```python
from build123d import *

# Parameters (mm, degrees)
F1_DEPTH = 7.5
F3_DEPTH = 5
F5_R     = 0.8
F6_DEPTH = 45


# Not quite as in the source:
# - ends of sketch curves that miss each other by under 0.0002 mm in the source are joined
# - a feature names something its author has since deleted; it is built from what else it names


with BuildPart() as f1:
    # F0 (on Right) → F1 (new body)
    with BuildSketch(Plane.YZ):
        with BuildLine():
            ThreePointArc((9.2226032736, 0.0929824566), (9.0820111575, -0.0673321366), (8.8773, -0.127))
            Line((8.8773, -0.127), (6.3627, -0.127))
            ThreePointArc((6.3627, -0.127), (6.1579888425, -0.0673321366), (6.0173967264, 0.0929824566))
            Line((6.0173967264, 0.0929824566), (5.6288146574, 0.9262855682))
            ThreePointArc((5.6288146574, 0.9262855682), (5.4882390894, 1.0842993961), (5.2850542, 1.143))
            Line((5.2850542, 1.143), (4.8749458, 1.143))
            ThreePointArc((4.8749458, 1.143), (4.668712979, 1.0823576494), (4.5281307776, 0.9197350317))
            Line((4.5281307776, 0.9197350317), (4.1426086033, 0.0929799713))
            ThreePointArc((4.1426086033, 0.0929799713), (4.0020111575, -0.0673321366), (3.7973, -0.127))
            Line((3.7973, -0.127), (1.2827, -0.127))
            ThreePointArc((1.2827, -0.127), (1.0779888425, -0.0673321366), (0.9373967264, 0.0929824566))
            Line((0.9373967264, 0.0929824566), (0.5488146574, 0.9262855682))
            ThreePointArc((0.5488146574, 0.9262855682), (0.4082390894, 1.0842993961), (0.2050542, 1.143))
            Line((0.2050542, 1.143), (-0.2050542, 1.143))
            ThreePointArc((-0.2050542, 1.143), (-0.411287021, 1.0823576494), (-0.5518692224, 0.9197350317))
            Line((-0.5518692224, 0.9197350317), (-0.9373913967, 0.0929799713))
            ThreePointArc((-0.9373913967, 0.0929799713), (-1.0779888425, -0.0673321366), (-1.2827, -0.127))
            Line((-1.2827, -0.127), (-3.7973, -0.127))
            ThreePointArc((-3.7973, -0.127), (-4.0020111575, -0.0673321366), (-4.1426032736, 0.0929824566))
            Line((-4.1426032736, 0.0929824566), (-4.5311853426, 0.9262855682))
            ThreePointArc((-4.5311853426, 0.9262855682), (-4.6717609106, 1.0842993961), (-4.8749458, 1.143))
            Line((-4.8749458, 1.143), (-5.2850542, 1.143))
            ThreePointArc((-5.2850542, 1.143), (-5.491287021, 1.0823576494), (-5.6318692224, 0.9197350317))
            Line((-5.6318692224, 0.9197350317), (-6.0173913967, 0.0929799713))
            ThreePointArc((-6.0173913967, 0.0929799713), (-6.1579888425, -0.0673321366), (-6.3627, -0.127))
            Line((-6.3627, -0.127), (-8.8773, -0.127))
            ThreePointArc((-8.8773, -0.127), (-9.0820111575, -0.0673321366), (-9.2226032736, 0.0929824566))
            Line((-9.2226032736, 0.0929824566), (-9.6111853426, 0.9262855682))
            ThreePointArc((-9.6111853426, 0.9262855682), (-9.7517609106, 1.0842993961), (-9.9549458, 1.143))
            Line((-9.9549458, 1.143), (-10.3650542, 1.143))
            ThreePointArc((-10.3650542, 1.143), (-10.571287021, 1.0823576494), (-10.7118692224, 0.9197350317))
            Line((-10.7118692224, 0.9197350317), (-11.0973913967, 0.0929799713))
            ThreePointArc((-11.0973913967, 0.0929799713), (-11.2379888425, -0.0673321366), (-11.4427, -0.127))
            Line((-11.4427, -0.127), (-12.7, -0.127))
            Line((-12.7, -0.127), (-12.7, -1.143))
            Line((-12.7, -1.143), (12.7, -1.143))
            Line((12.7, -1.143), (12.7, -0.127))
            Line((12.7, -0.127), (11.4427, -0.127))
            ThreePointArc((11.4427, -0.127), (11.2379888425, -0.0673321366), (11.0973967264, 0.0929824566))
            Line((11.0973967264, 0.0929824566), (10.7088146574, 0.9262855682))
            ThreePointArc((10.7088146574, 0.9262855682), (10.5682390894, 1.0842993961), (10.3650542, 1.143))
            Line((10.3650542, 1.143), (9.9549458, 1.143))
            ThreePointArc((9.9549458, 1.143), (9.748712979, 1.0823576494), (9.6081307776, 0.9197350317))
            Line((9.6081307776, 0.9197350317), (9.2226032736, 0.0929824566))
        make_face()
    extrude(amount=-F1_DEPTH)

    # F2 (on face) → F3 (join)
    with BuildSketch(Plane(origin=(-7.5, 0, 0), x_dir=(0, -1, 0), z_dir=(-1, 0, 0))):
        Polygon((-11.4427, -0.127), (-12.7, -0.127), (-12.7, -1.143), (12.7, -1.143), (12.7, -0.127), (11.4427, -0.127), (8.8773, -0.127), (6.3627, -0.127), (3.7973, -0.127), (1.2827, -0.127), (-1.2827, -0.127), (-3.7973, -0.127), (-6.3627, -0.127), (-8.8773, -0.127), align=None)
    extrude(amount=F3_DEPTH)

    # F4: F1 across plane


with BuildPart() as f1_1:
    add(f1.part)
    add(f1.part.mirror(Plane.YZ))

    # F5 (on face) → F6 (cut)
    with BuildSketch(Plane.XY.offset(-0.127)):
        with Locations((10, 7.7)):
            Circle(F5_R)
        with Locations((10, -7.7)):
            Circle(F5_R)
        with Locations((-10, 7.7)):
            Circle(F5_R)
        with Locations((-10, -7.7)):
            Circle(F5_R)
    extrude(amount=-F6_DEPTH, mode=Mode.SUBTRACT)


solid = f1_1.part
```
Could you check a few things on this model? Use its own coordinates, in mm. A direction names the side the tool comes from. Give positions to 0.01 mm unless a question says otherwise; leave off trailing zeros. Write each loop counter-clockwise with the first axis right and the second up, starting at its lowest first coordinate (ties: lowest second). Pieces come first, ordered by that corner, then holes. Notation, with made-up numbers: (47, 20) - (91, 20) arc R12 ccw to (91, 29) - close; hole circle Ø8 at (48, -8.75). An arc over 180 degrees is marked (long way). One line per item, written item: value. Start each with the question number.
Item 1: Please list where these lines run through material, in increasing order: line 1 (Y direction, x = -10, z = -0.7); line 2 (Y direction, x = 7, z = 0.25); line 3 (Z direction, x = -10.25, y = -6.5). Write a range as from..to.
Item 2: Imagine slicing it at C-C, the plane z = 0.4. List the corners of the cut face in (x, y) for me.
Item 3: Imagine slicing it at B-B, the plane x = 10. List the corners of the cut face in (y, z) for me, and give its area (3 significant figures).
Item 4: Imagine slicing it at A-A, the plane y = 7.7. List the corners of the cut face in (x, z) for me, and give its area (3 significant figures).
Item 5: Which directions (+Z, -Z, +X, -X, +Y, -Y) give clear straight access to the entire face, cutting with the end or side of a thin tool? Please do faces 5 (the face through (-0.105, 9.418, 0.512)), 6 (the face through (-0.105, 10.906, 0.504)), 7 (the face through (-7.5, 5.1, 0.4)), 8 (the face through (7.5, 5.1, 0.4)).
Item 6: If we mould it in two halves opening along Y, with no side actions, what happens to faces 1 (the face through (9.37, 7.21, -0.63)), 2 (the face through (-0.2, 12.7, -0.6)), 3 (the face through (-0.105, 5.826, 0.504)), 4 (the face through (-7.5, -5.1, 0.4))? For each: +Y half, -Y half, draft (parallel to the pull), parting line (faces both ways), or undercut.
Item 7: I'm going to push flat-ended pins straight in: pin 1 (1 mm diameter, centred on y = -5.5, z = 0.5, fed in from +X); pin 2 (1.8 mm diameter, centred on x = 10, y = -7.7, fed in from +Z); pin 3 (0.6 mm diameter, centred on y = 0, z = 1, fed in from -X); pin 4 (7.5 mm diameter, centred on x = 1, y = -2.5, fed in from +Z). Where does each tip first touch, or does it pass through?
Geometry says:
1. line 1: -12.7..-8.5, -6.9..6.9, 8.5..12.7
1. line 2: -11.02..-9.3, -5.94..-4.22, -0.86..0.86, 4.22..5.94, 9.3..11.02
1. line 3: -1.14..-0.13
2. outline: (-7.5, -10.95) - (7.5, -10.95) - (7.5, -9.37) - (-7.5, -9.37) - close; (-7.5, -5.87) - (7.5, -5.87) - (7.5, -4.29) - (-7.5, -4.29) - close; (-7.5, -0.79) - (7.5, -0.79) - (7.5, 0.79) - (-7.5, 0.79) - close; (-7.5, 4.29) - (7.5, 4.29) - (7.5, 5.87) - (-7.5, 5.87) - close; (-7.5, 9.37) - (7.5, 9.37) - (7.5, 10.95) - (-7.5, 10.95) - close
3. outline: (-12.7, -1.14) - (-8.5, -1.14) - (-8.5, -0.13) - (-12.7, -0.13) - close; (-6.9, -1.14) - (6.9, -1.14) - (6.9, -0.13) - (-6.9, -0.13) - close; (8.5, -1.14) - (12.7, -1.14) - (12.7, -0.13) - (8.5, -0.13) - close
3. area: 22.6 mm^2
4. outline: (-12.5, -1.14) - (-10.8, -1.14) - (-10.8, -0.13) - (-12.5, -0.13) - close; (-9.2, -1.14) - (9.2, -1.14) - (9.2, -0.13) - (-9.2, -0.13) - close; (10.8, -1.14) - (12.5, -1.14) - (12.5, -0.13) - (10.8, -0.13) - close
4. area: 22.1 mm^2
5. face 5: +Z, +X, -X
5. face 6: +Z, +X, -X, +Y
5. face 7: +Z, -X, +Y, -Y
5. face 8: +Z, +X, +Y, -Y
6. face 1: undercut
6. face 2: +Y half
6. face 3: undercut
6. face 4: draft
7. pin 1: x = 7.5
7. pin 2: z = -0.13
7. pin 3: x = -7.5
7. pin 4: z = 1.14
